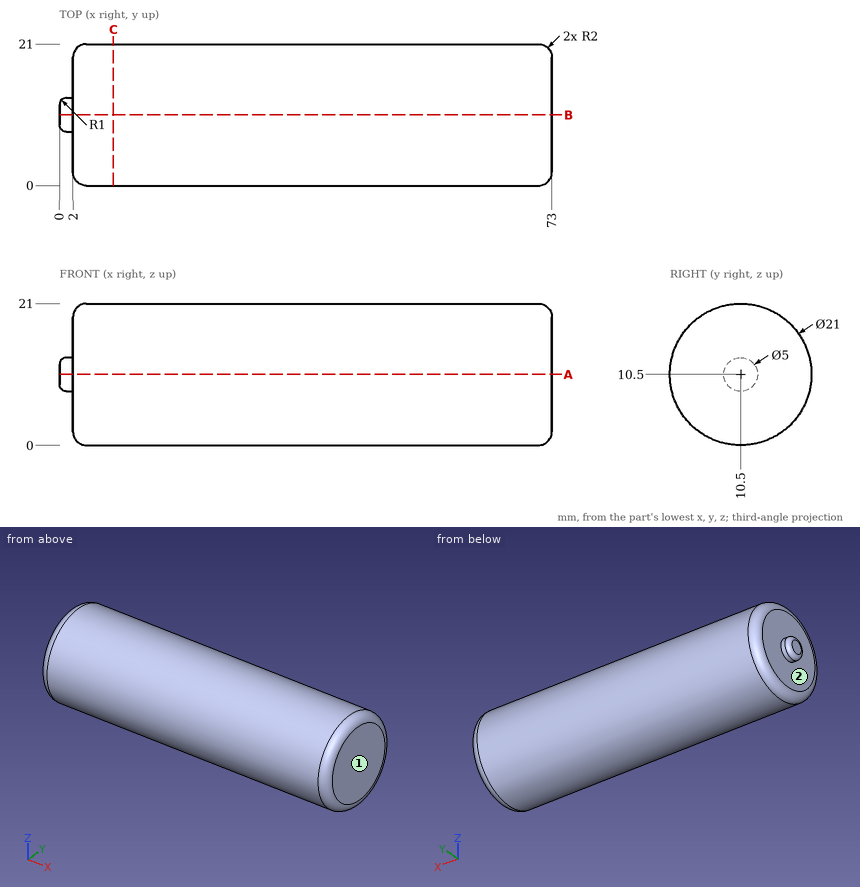
Design review of the part shown in the three views and the two pictorial views. Dimensions are in mm from the part's minimum x, y and z. A direction names the side the tool comes from. Coordinates: 2 decimals unless noted, no trailing zeros. Order: outer loops, then holes, each group sorted by start corner. A loop starts at its lowest first (then second) coordinate and runs counter-clockwise, first axis right, second up.
1) Clearance check with flat-ended pins moving along their axes: pin 1 (8 mm diameter, centred on y = 12, z = 3.5, fed in from -X); pin 2 (12 mm diameter, centred on y = 10, z = 18, fed in from -X); pin 3 (5 mm diameter, centred on x = 11.5, z = 2, fed in from -Y); pin 4 (1 mm diameter, centred on x = 33.5, y = 3, fed in from +Z). State where each tip first meets the part, or that it passes through.
2) For the marked faces 1 and 2, list the 3-axis set-ups (+Z, -Z, +X, -X, +Y, -Y) from which the entire face can be reached by the end or side of a thin tool; tool diameter is ignored.
3) Wall thickness on line 1 along X through (y, z) = (7.25, 18); line 2 along Z through (x, y) = (8.5, 11); line 3 along Z through (x, y) = (64.5, 7): over which ranges is each line inside the solid? List them lowest first.
4) Take a section at C-C, the plane x = 8. Give the boundary of the cut face in (y, z), and give its area (3 significant figures).
5) Take a section at A-A, the plane z = 10.5. Give the boundary of the cut face in (x, y), and give its area (3 significant figures).
Returned:
1. pin 1: stops at x = 2
1. pin 2: stops at x = 0
1. pin 3: stops at y = 1.88
1. pin 4: stops at z = 18.33
2. face 1: +Z, -Z, +X, +Y, -Y
2. face 2: -X
3. line 1: x = 2 to 73
3. line 2: z = 0.01 to 20.99
3. line 3: z = 0.6 to 20.4
4. outline: circle Ø21 at (10.5, 10.5)
4. area: 346 mm2
5. outline: (0, 9) arc R1 ccw to (1, 8) - (2, 8) - (2, 2) arc R2 ccw to (4, 0) - (71, 0) arc R2 ccw to (73, 2) - (73, 19) arc R2 ccw to (71, 21) - (4, 21) arc R2 ccw to (2, 19) - (2, 13) - (1, 13) arc R1 ccw to (0, 12) - close
5. area: 1,500 mm2
